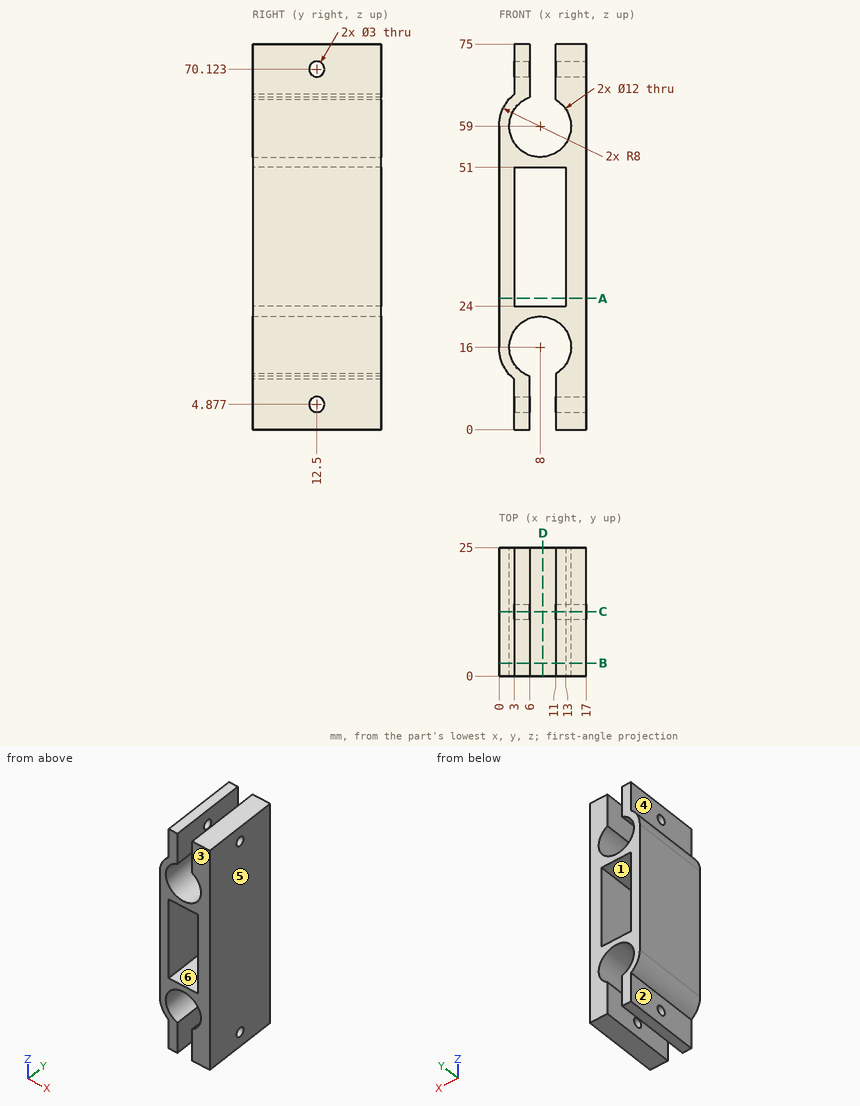
Geometry: see drawing. Coordinates: mm, zero at the bounding-box minimum. A direction names the side the tool comes from. Give positions to 0.01 mm unless a question says otherwise; leave off trailing zeros. Order: outer loops, then holes, each group sorted by start corner. A loop starts at its lowest first (then second) coordinate and runs counter-clockwise, first axis right, second up. Notation, with made-up numbers: M 13,71 L 67,71 A25 cw 67,95 Z; hole C -8,68.25 d4. An arc over 180 degrees is marked long. Answer as CSV lines item,"result". Start each with the question number.
1) Mould query, pull axis X, two halves, no side actions, for the marked faces 1, 2 and 3. Classes: +X half, -X half, draft (parallel to the pull), parting line (faces both ways), or undercut.
2) Cut plane C-C (y = 12.5). State how many separate pieces and enclosed holes the cut face has, then the cut area to 3 significant figures.
3) Set-up query: the marked faces 4, 5 and 6. Return all of +Z, -Z, +X, -X, +Y, -Y with unobstructed straight access to the full face (end or side cutting, diameter ignored); none if empty.
4) Line query: line 1 (Z direction, x = 15.6, y = 12.5); line 2 (X direction, y = 10, z = 27); line 3 (X direction, y = 11.5, z = 7). Output: solid intervals per line, ascending. Write a range as from..to.
5) Cut plane D-D (x = 8.5). Output: boundary loops of the cut face in (y, z), then the cut area to 3 significant figures.
6) First-contact query: P1, Ø3.5, axis at y = 12.5, z = 4.88, coming from the -X side; P2, Ø5, axis at x = 6, z = 14, coming from the +Y side. Flat tips, straight axial feed; report the tip coordinate or a pass-through.
7) Cut plane B-B (y = 2.5). Output: boundary loops of the cut face in (x, z) (1 decimal).
8) Cut plane A-A (z = 25.5). Output: boundary loops of the cut face in (x, y), then the cut area to 3 significant figures.
Findings below:
1,face 1,"undercut"
1,face 2,"-X half"
1,face 3,"draft"
2,separate pieces,"5"
2,enclosed holes,"1"
2,area,"553 mm²"
3,face 4,"+Z, -X, +Y, -Y"
3,face 5,"+Z, -Z, +X, +Y, -Y"
3,face 6,"+Y, -Y"
4,line 1,"z = 0..3.38, 6.38..68.62, 71.62..75"
4,line 2,"x = 0..3, 13..17"
4,line 3,"x = 3..6, 11..17"
5,outline,"M 0,21.98 L 25,21.98 L 25,24 L 0,24 Z; M 0,51 L 25,51 L 25,53.02 L 0,53.02 Z"
5,area,"101 mm²"
6,P1,"stops at x = 3"
6,P2,"passes through"
7,outline,"M 0,16 A8 ccw 3,9.8 L 3,0 L 6,0 L 6,10.3 A6 cw long 11,10.8 L 11,0 L 17,0 L 17,75 L 11,75 L 11,64.2 A6 cw long 6,64.7 L 6,75 L 3,75 L 3,65.2 A8 ccw 0,59 Z; hole M 3,24 L 13,24 L 13,51 L 3,51 Z"
8,outline,"M 0,0 L 3,0 L 3,25 L 0,25 Z; M 13,0 L 17,0 L 17,25 L 13,25 Z"
8,area,"175 mm²"
